For this review, use the dimensioned drawing (mm, ordinates from the lowest corner) and the shaded views. A direction names the side the tool comes from. Give positions to 0.01 mm unless a question says otherwise; leave off trailing zeros. Order: outer loops, then holes, each group sorted by start corner. A loop starts at its lowest first (then second) coordinate and runs counter-clockwise, first axis right, second up.
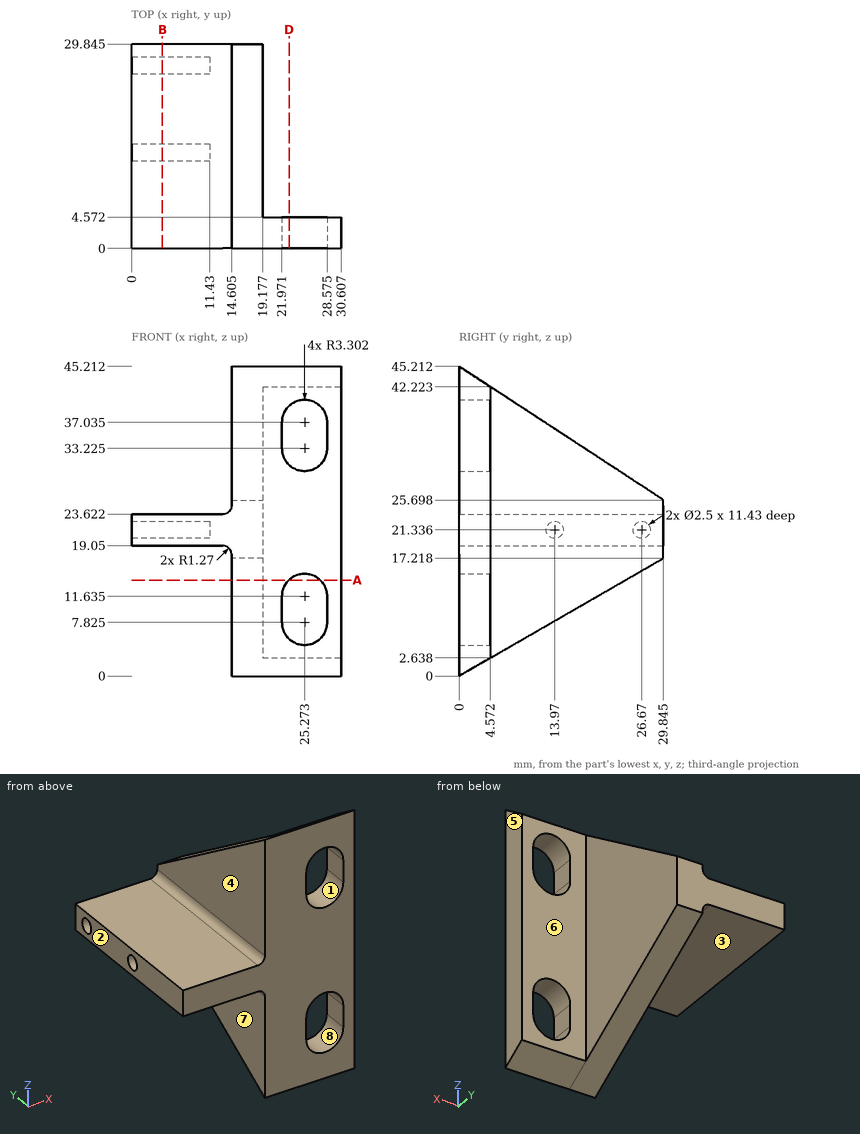
1. To check wall thickness, follow line 1 (X direction, y = 1, z = 8.5) (1 decimal); line 2 (X direction, y = 23.75, z = 27.5) (1 decimal); line 3 (X direction, y = 18.25, z = 20). State the ranges of each line that lie inside material, in increasing order.
2. Draft analysis for pull direction X (two halves, no side actions). For the marked faces 1, 2 and 3, state which applies: pulls with the +X half, pulls with the -X half, needs draft (parallel to the pull), parting line crosses it, or undercut.
3. For the marked faces 4, 5, 6, 7 and 8, list the 3-axis set-ups (+Z, -Z, +X, -X, +Y, -Y) from which the entire face can be reached by the end or side of a thin tool; tool diameter is ignored.
4. Take a section at B-B (x = 4.5). Count the separate pieces of the cut face and the enclosed holes in it, and give its area (3 significant figures).
5. Take a section at D-D (x = 23). Write out the cut boundary in (y, z).
6. Take a section at A-A (z = 14). Write out the cut boundary in (x, y) (1 decimal).
7. Insertion check: pin 1 (3 mm diameter, centred on x = 8.5, y = 23.5, fed in from +Z); pin 2 (3 mm diameter, centred on y = 13.97, z = 21.336, fed in from -X); pin 3 (4 mm diameter, centred on x = 9.5, y = 12.5, fed in from -Z); pin 4 (5.5 mm diameter, centred on x = 23, z = 19, fed in from +Y). Each pin has a flat end and moves straight along its axis. Give the tip position at first contact, or say it passes through.
Answer:
1. line 1: x = 14.6 to 22, 28.6 to 30.6
1. line 2: x = 14.6 to 19.2
1. line 3: x = 0 to 19.18
2. face 1: undercut
2. face 2: pulls with the -X half
2. face 3: needs draft
3. face 4: +Z, -X, +Y, -Y
3. face 5: +Z, -Z, +X, +Y, -Y
3. face 6: +Z, -Z, +X, +Y
3. face 7: -Z, -X, +Y, -Y
3. face 8: +Y, -Y
4. separate pieces: 1
4. enclosed holes: 2
4. area: 127 mm2
5. outline: (0, 0) - (4.57, 2.64) - (4.57, 5.43) - (0, 5.43) - close; (0, 14.03) - (4.57, 14.03) - (4.57, 30.83) - (0, 30.83) - close; (0, 39.43) - (4.57, 39.43) - (4.57, 42.22) - (0, 45.21) - close
6. outline: (14.6, 0) - (23, 0) - (23, 4.6) - (19.2, 4.6) - (19.2, 24.3) - (14.6, 24.3) - close; (27.6, 0) - (30.6, 0) - (30.6, 4.6) - (27.6, 4.6) - close
7. pin 1: stops at z = 23.62
7. pin 2: stops at x = 0
7. pin 3: stops at z = 19.05
7. pin 4: stops at y = 4.57
